Here's how the part is built. I have some questions about the finished solid (model axes, mm). A direction names the side the tool comes from. Round coordinates to 2 decimals unless told otherwise and drop trailing zeros. Write each loop counter-clockwise with the first axis right and the second up, starting at its lowest first coordinate (ties: lowest second). Pieces come first, ordered by that corner, then holes. Notation, with made-up numbers: M -35.75,88 L -5.75,88 A22 ccw -5.75,110 Z; hole C 37.25,-18.5 d4. An arc over 180 degrees is marked long. Use a Markdown table: item, result. Add a question column.
Autodesk Inventor part; units mm, degrees
ref_plane "YZ Plane" through (0, 0, 0) normal (1, 0, 0) x (0, 1, 0)
ref_plane "XZ Plane" through (0, 0, 0) normal (0, 1, 0) x (-1, 0, 0)
ref_plane "XY Plane" through (0, 0, 0) normal (0, 0, 1) x (1, 0, 0)
sketch "Sketch1" plane through (0, 0, 0) normal (0, 0, 1) x (1, 0, 0)
  line L0 (0, 0) -> (70, 0)
  line L1 (70, 0) -> (70, 70)
  line L2 (70, 70) -> (0, 70)
  line L3 (0, 70) -> (0, 0)
  dimension "d0" = 70
  dimension "d1" = 70
extrude "Extrusion1" add sketch "Sketch1" along normal blind 3
sketch "Esboço3" plane through (0, 0, 3) normal (0, 0, 1) x (1, 0, 0)
  line L0 (70, 70) -> (0, 70)
  line L1 (70, 0) -> (70, 70)
  line L2 (0, 70) -> (0, 0)
  line L3 (41, 63) -> (29, 63)
  line L4 (29, 63) -> (29, 38)
  line L5 (29, 38) -> (41, 38)
  line L6 (41, 38) -> (41, 63)
  line L7 (41, 7) -> (29, 7)
  line L8 (29, 7) -> (29, 32)
  line L9 (29, 32) -> (41, 32)
  line L10 (41, 32) -> (41, 7)
  line L11 (0, 0) -> (70, 0)
  circle A0 centre (23, 19.5) radius 1.5
  circle A1 centre (23, 19.5) radius 4.5
  circle A2 centre (47, 19.5) radius 1.5
  circle A3 centre (47, 19.5) radius 4.5
  circle A4 centre (23, 50.5) radius 4.5
  circle A5 centre (23, 50.5) radius 1.5
  circle A6 centre (47, 50.5) radius 1.5
  circle A7 centre (47, 50.5) radius 4.5
  line L12 (18.5, 7) -> (51.5, 7)
  line L13 (51.5, 7) -> (51.5, 63)
  line L14 (51.5, 63) -> (18.5, 63)
  line L15 (18.5, 63) -> (18.5, 7)
  point P0 (35, 70)
  point P1 (35, 63)
  point P2 (35, 7)
  point P3 (29, 50.5)
  point P4 (35, 32)
  point P5 (18.5, 50.5)
  point P6 (18.5, 19.5)
  point P7 (51.5, 19.5)
  point P8 (51.5, 50.5)
  dimension "d10" = 70
  dimension "d11" = 12
  dimension "d12" = 25
  dimension "d13" = 7
  dimension "d14" = 35
  dimension "d15" = 12
  dimension "d16" = 25
  dimension "d17" = 7
  dimension "d18" = 35
  dimension "d21" = 3
  dimension "d22" = 12.5
  dimension "d24" = 9
  dimension "d25" = 6
  dimension "d26" = 3
  dimension "d27" = 9
  dimension "d28" = 6
  dimension "d29" = 12.5
  dimension "d30" = 9
  dimension "d31" = 6
  dimension "d32" = 3
  dimension "d33" = 12.5
  dimension "d34" = 3
  dimension "d35" = 9
  dimension "d36" = 12.5
  dimension "d37" = 6
  dimension "d40" = 56
  dimension "d41" = 16.5
  dimension "d42" = 16.5
extrude "Extrusão4" add sketch "Esboço3" along normal blind 9 contours L6 L5 L4 L3 | A4 | A1 | A3 | A7 | L14 L13 L12 L10 L9 L8 L15 L4 L5 L6 | L7 L8 L9 L10
sketch "Esboço4" plane through (0, 0, 12) normal (0, 0, 1) x (1, 0, 0)
  line L0 (70, 70) -> (0, 70)
  line L1 (70, 0) -> (70, 70)
  line L2 (0, 70) -> (0, 0)
  line L3 (41, 63) -> (29, 63)
  line L4 (29, 63) -> (29, 38)
  line L5 (29, 38) -> (41, 38)
  line L6 (41, 38) -> (41, 63)
  line L7 (41, 7) -> (29, 7)
  line L8 (29, 7) -> (29, 32)
  line L9 (29, 32) -> (41, 32)
  line L10 (41, 32) -> (41, 7)
  line L11 (0, 0) -> (70, 0)
  circle A0 centre (23, 19.5) radius 1.5
  circle A1 centre (23, 19.5) radius 4.5
  circle A2 centre (47, 19.5) radius 1.5
  circle A3 centre (47, 19.5) radius 4.5
  circle A4 centre (23, 50.5) radius 4.5
  circle A5 centre (23, 50.5) radius 1.5
  circle A6 centre (47, 50.5) radius 1.5
  circle A7 centre (47, 50.5) radius 4.5
  line L12 (18.5, 7) -> (51.5, 7)
  line L13 (51.5, 7) -> (51.5, 63)
  line L14 (51.5, 63) -> (18.5, 63)
  line L15 (18.5, 63) -> (18.5, 7)
  point P0 (35, 70)
  point P1 (35, 63)
  point P2 (35, 7)
  point P3 (29, 50.5)
  point P4 (35, 32)
  point P5 (18.5, 50.5)
  point P6 (18.5, 19.5)
  point P7 (51.5, 19.5)
  point P8 (51.5, 50.5)
  dimension "d43" = 70
  dimension "d44" = 12
  dimension "d45" = 25
  dimension "d46" = 7
  dimension "d47" = 35
  dimension "d48" = 12
  dimension "d49" = 25
  dimension "d50" = 7
  dimension "d51" = 35
  dimension "d52" = 3
  dimension "d53" = 12.5
  dimension "d54" = 9
  dimension "d55" = 6
  dimension "d56" = 3
  dimension "d57" = 9
  dimension "d58" = 6
  dimension "d59" = 12.5
  dimension "d60" = 9
  dimension "d61" = 6
  dimension "d62" = 3
  dimension "d63" = 12.5
  dimension "d64" = 3
  dimension "d65" = 9
  dimension "d66" = 12.5
  dimension "d67" = 6
  dimension "d68" = 56
  dimension "d69" = 16.5
  dimension "d70" = 16.5
extrude "Extrusão5" cut sketch "Esboço4" against normal blind 2 contours L6 L5 L4 L3 | L7 L8 L9 L10
sketch "Esboço5" plane through (0, 0, 3) normal (0, 0, 1) x (1, 0, 0)
  line L0 (0, 0) -> (70, 0)
  line L1 (10, 0) -> (60, 0)
  line L2 (60, 0) -> (60, 7)
  line L3 (60, 7) -> (10, 7)
  line L4 (10, 7) -> (10, 0)
  line L5 (70, 70) -> (0, 70)
  line L6 (10, 70) -> (60, 70)
  line L7 (60, 70) -> (60, 63)
  line L8 (60, 63) -> (10, 63)
  line L9 (10, 63) -> (10, 70)
  point P0 (35, 0)
  point P1 (60, 3.5)
  point P2 (10, 66.5)
  point P3 (35, 70)
  dimension "d73" = 50
  dimension "d74" = 25
  dimension "d75" = 7
  dimension "d76" = 50
  dimension "d77" = 7
  dimension "d78" = 25
extrude "Extrusão6" cut sketch "Esboço5" against normal up to surface (3 mm away)
sketch "Esboço6" plane through (0, 0, 3) normal (0, 0, 1) x (1, 0, 0)
  circle A0 centre (-25, 35) radius 35
  line L0 (0, 70) -> (0, 0)
  line L1 (0, 0) -> (10, 0)
  circle A1 centre (95, 35) radius 35
  line L2 (70, 0) -> (70, 70)
  line L3 (60, 0) -> (70, 0)
  circle A2 centre (4, 66) radius 1.75
  circle A3 centre (66, 66) radius 1.75
  circle A4 centre (4, 4) radius 1.75
  circle A5 centre (66, 4) radius 1.75
  line L4 (10, 70) -> (0, 70)
  line L5 (70, 70) -> (60, 70)
  circle A6 centre (14.5, 35) radius 1.75
  line L6 (18.5, 63) -> (18.5, 7)
  circle A7 centre (55.5, 35) radius 1.75
  line L7 (51.5, 7) -> (51.5, 63)
  point P0 (0, 35)
  point P1 (65, 0)
  point P2 (70, 10.5051)
  point P3 (70, 59.4949)
  point P4 (0, 59.4949)
  point P5 (0, 10.5051)
  dimension "d81" = 70
  dimension "d82" = 25
  dimension "d83" = 35
  dimension "d84" = 70
  dimension "d85" = 25
  dimension "d86" = 35
  dimension "d89" = 3.5
  dimension "d90" = 3.5
  dimension "d91" = 3.5
  dimension "d92" = 3.5
  dimension "d93" = 4
  dimension "d94" = 4
  dimension "d95" = 4
  dimension "d96" = 4
  dimension "d97" = 4
  dimension "d98" = 4
  dimension "d99" = 4
  dimension "d100" = 4
  dimension "d101" = 3.5
  dimension "d102" = 4
  dimension "d103" = 35
  dimension "d104" = 3.5
  dimension "d105" = 4
  dimension "d106" = 35
extrude "Extrusão7" cut sketch "Esboço6" against normal up to surface (3 mm away) contours A0 L0 | L2 A1 | A2 | A3 | A4 | A5 | A6 | A7 picked at (1.4165, 28.5928) picked at (66.7381, 33.7107)
sketch "Esboço7" plane through (0, 0, 3) normal (0, 0, 1) x (1, 0, 0)
  point P0 (0, 0)
equation "\"d30\" = d24"
equation "\"d32\" = d21"
equation "\"d33\" = d22"
equation "\"d34\" = d21"
equation "\"d35\" = d27"
equation "\"d36\" = d29"
equation "\"d37\" = d28"
equation "\"d60\" = d54"
equation "\"d62\" = d52"
equation "\"d63\" = d53"
equation "\"d64\" = d52"
equation "\"d65\" = d57"
equation "\"d66\" = d59"
equation "\"d67\" = d58"
equation "\"d90\" = d89"
Item 1: Imagine slicing it at B-B on x = 14.5. List the corners of the cut face in (y, z) for me.
Item 2: Imagine slicing it at C-C on z = 7.5. List the corners of the cut face in (x, y) for me.
Item 3: On a 3-axis mill with a long thin cutter (end or side, diameter ignored), from which of +Z, -Z, +X, -X, +Y, -Y can I reach the whole of each face in a straight line? I mean faces 1 (the face through (35, 20, 10)), 2 (the face through (47, 20, 3)), 3 (the face through (35, 38, 11)). Say none if no direction works.
Item 4: Imagine slicing it at A-A on y = 4. List the corners of the cut face in (x, z) for me.
Item 5: I need wall thicknesses on probe 1 along Y at (x, z) = (23, 6.25); probe 2 along X at (y, z) = (66, 2.1); probe 3 along X at (y, z) = (6, 1). Which ranges of each line are inside material? Lowest first, please. Write a range as from..to.
Item 6: For pin 1 Ø3.5 at (x, y) = (33.5, 25.5) entering from +Z; pin 2 Ø0.9 at (x, y) = (47.5, 50) entering from +Z; pin 3 Ø4 at (y, z) = (25.5, 1.5) entering from -X, each with a flat end and sliding along its axis, tell me the tip position at first contact or that it passes through.
Item 7: Imagine slicing it at D-D on z = 2. List the corners of the cut face in (x, y) for me, plus the area to 3 significant figures.
Item 8: If we mould it in two halves opening along X, with no side actions, what happens to faces 4 (the face through (35, 32, 11)), 5 (the face through (10, 35, 2)), 6 (the face through (10, 4, 2)), 7 (the face through (35, 35, 12))? For each: +X half, -X half, draft (parallel to the pull), parting line (faces both ways), or undercut.
The answers:
| question | item | result |
|---|---|---|
| 1 | outline | M 7,0 L 33.25,0 L 33.25,3 L 7,3 Z; M 36.75,0 L 63,0 L 63,3 L 36.75,3 Z |
| 2 | outline | M 18.5,7 L 51.5,7 L 51.5,63 L 18.5,63 Z; hole C 23,19.5 d3; hole C 23,50.5 d3; hole C 47,19.5 d3; hole C 47,50.5 d3 |
| 3 | face 1 | +Z, -Y |
| 3 | face 2 | +Z |
| 3 | face 3 | +Z, +Y |
| 4 | outline | M 0,0 L 2.25,0 L 2.25,3 L 0,3 Z; M 5.75,0 L 10,0 L 10,3 L 5.75,3 Z; M 60,0 L 64.25,0 L 64.25,3 L 60,3 Z; M 67.75,0 L 70,0 L 70,3 L 67.75,3 Z |
| 5 | probe 1 | 7..18, 21..49, 52..63 |
| 5 | probe 2 | 0..2.25, 5.75..10, 60..64.25, 67.75..70 |
| 5 | probe 3 | 0..10, 60..70 |
| 6 | pin 1 | z = 10 |
| 6 | pin 2 | z = 3 |
| 6 | pin 3 | x = 8.06 |
| 7 | outline | M 0,0 L 10,0 L 10,7 L 60,7 L 60,0 L 70,0 L 70,10.51 A35 cw 70,59.49 L 70,70 L 60,70 L 60,63 L 10,63 L 10,70 L 0,70 L 0,59.49 A35 cw 0,10.51 Z; hole C 4,4 d3.5; hole C 4,66 d3.5; hole C 14.5,35 d3.5; hole C 55.5,35 d3.5; hole C 66,4 d3.5; hole C 66,66 d3.5 |
| 7 | area | 3,470 mm² |
| 8 | face 4 | undercut |
| 8 | face 5 | -X half |
| 8 | face 6 | undercut |
| 8 | face 7 | draft |
